from build123d import *

# Parameters (mm, degrees)
SKETCH1_R           = 12.3
SKETCH1_R_2         = 11.9
SKETCH1_R_3         = 10.3
SKETCH1_R_4         = 10.95
SKETCH1_R_5         = 12.35
SKETCH1_R_6         = 9
BOSS_EXTRUDE4_DEPTH = 59
SKETCH4_R           = 8.15
SKETCH4_R_2         = 11.5
SKETCH4_R_3         = 10.1
SKETCH4_R_4         = 11.45
SKETCH4_R_5         = 9.45
SKETCH4_R_6         = 11.05
CUT_EXTRUDE2_DEPTH  = 57
BOSS_EXTRUDE5_DEPTH = 2


with BuildPart() as part:
    # Sketch1 → Boss-Extrude4 (new body)
    with BuildSketch(Plane(origin=(0, 0, 0), x_dir=(1, 0, 0), z_dir=(0, 1, 0))):
        with Locations((35.512781465, 27.639016147)):
            Circle(SKETCH1_R)
        with Locations((36.005267937, -1.447561772)):
            Circle(SKETCH1_R_2)
        with Locations((51.661033243, 13.068619292)):
            Circle(SKETCH1_R_3)
        with Locations((18.919707674, 12.591428229)):
            Circle(SKETCH1_R_4)
        with Locations((6.200754384, 31.090907335)):
            Circle(SKETCH1_R_5)
        with Locations((22.571970647, 43.529254056)):
            Circle(SKETCH1_R_6)
    extrude(amount=BOSS_EXTRUDE4_DEPTH)

    # Sketch4 → Cut-Extrude2 (cut)
    with BuildSketch(Plane(origin=(0, 59, 0), x_dir=(1, 0, 0), z_dir=(0, 1, 0))):
        with Locations(Location((22.611280457, 43.589861599, 0), (0, 0, 270))):
            Circle(SKETCH4_R)
        with Locations(Location((6.240064194, 31.151514878, 0), (0, 0, 270))):
            Circle(SKETCH4_R_2)
        with Locations(Location((18.959017484, 12.652035772, 0), (0, 0, 270))):
            Circle(SKETCH4_R_3)
        with Locations(Location((35.552091275, 27.69962369, 0), (0, 0, 270))):
            Circle(SKETCH4_R_4)
        with Locations(Location((51.700343053, 13.129226835, 0), (0, 0, 270))):
            Circle(SKETCH4_R_5)
        with Locations(Location((36.044577747, -1.386954229, 0), (0, 0, 270))):
            Circle(SKETCH4_R_6)
    extrude(amount=-CUT_EXTRUDE2_DEPTH, mode=Mode.SUBTRACT)

    # Sketch5 → Boss-Extrude5 (add)
    with BuildSketch(Plane(origin=(0, 59, 0), x_dir=(1, 0, 0), z_dir=(0, 1, 0))):
        Polygon((40.81243907, -1.58402798), (51.520532369, 9.252965923), (56.778337624, 3.7224031), (58.688878923, 5.538719884), (16.370888419, 50.052027945), (14.460347121, 48.235711161), (17.926333207, 44.589921166), (6.147145479, 32.668939341), (-1.681518051, 40.404484846), (-3.988115938, 38.070120871), (44.470030089, -9.811639827), (46.776627976, -7.477275852), align=None)
        Polygon((36.463308943, 25.091308361), (47.227733247, 13.768461283), (36.382771282, 2.792951133), (25.275141449, 13.768461283), align=None, mode=Mode.SUBTRACT)
        Polygon((21.642995472, 40.680450739), (32.86204414, 28.879394887), (21.559056386, 17.440345379), (9.982307257, 28.879394887), align=None, mode=Mode.SUBTRACT)
    extrude(amount=BOSS_EXTRUDE5_DEPTH)


solid = part.part
Build history of the part. All positions in model axes, mm. A direction names the side the tool comes from. Coordinates: 2 decimals unless noted, no trailing zeros. Order: outer loops, then holes, each group sorted by start corner. A loop starts at its lowest first (then second) coordinate and runs counter-clockwise, first axis right, second up. Notation, with made-up numbers: (41.25, 0.5) - (48.25, 0.5) arc R21 cw to (48.25, 33.5) - close; hole circle Ø8 at (-17, -15.5). An arc over 180 degrees is marked (long way). Write item = value, one per line. Start each with the question number.
1) Wall check: line 1 along X through (y, z) = (26.5, -37); line 2 along X through (y, z) = (35, -40.5); line 3 along X through (y, z) = (6, -15). Give the ranges that are in metal, low to high. Write a range as from..to.
2) 3-axis set-ups, long thin cutter, end or side, ignore diameter. For faces 4 (the face through (15.85, 59.99, -23.08)), 5 (the face through (44, 59, -36)), 6 (the face through (19.902, 59.986, -14.464)): which of +Z, -Z, +X, -X, +Y, -Y reach the whole face in a straight line?
3) Saw through at C-C on y = 36. Count the separate pieces of the cut face and the enclosed holes in it, then the cut area to 3 significant figures.
4) Saw through at B-B on x = 50. Write the cut outline in (y, z) (3 decimals).
5) Two-plate mould, pull along X, no slides. Class faces 1 (the face through (10.788, 29.087, -5.258)), 2 (the face through (57.7, 60, -4.6)), 3 (the face through (14, 59, -44)): pulls with the +X half, pulls with the -X half, needs draft (parallel to the pull), parting line crosses it, or undercut.
6) Saw through at A-A on z = -12.5. Write the cut outline in (x, y), then the cut area to 3 significant figures.
7) Saw through at D-D on x = 34.5. Write the cut outline in (y, z), then the cut area to 3 significant figures.
8) Flat gauge pins, fed straight in: pin 1 Ø15 at (x, z) = (21, -2.5) entering from +Y; pin 2 Ø3 at (y, z) = (11, -14) entering from -X; pin 3 Ø6 at (x, z) = (23, -21.5) entering from -Y; pin 4 Ø6 at (x, y) = (13, 47.5) entering from +Z. Where does each tip first touch, or does it go through?
From the geometry:
q1.line_1 = -4.64..-3.66, 16.14..17.82, 27.41..28.87, 42.23..43.49
q1.line_2 = -1.8..-0.46, 12.94..15.07, 30.15..31.05
q1.line_3 = 8.24..9.14, 28.78..29.6, 41.54..42.44, 60.96..61.78
q2.face_4 = +Y
q2.face_5 = -Z, +X, +Y
q2.face_6 = +Z, -X, +Y
q3.separate_pieces = 1
q3.enclosed_holes = 8
q3.area = 320 mm^2
q4.outline = (0, -23.234) - (59, -23.234) - (59, -22.425) - (2, -22.425) - (2, -3.833) - (59, -3.833) - (59, -2.903) - (0, -2.903) - close; (59, -14.678) - (61, -14.678) - (61, -7.714) - (59, -7.714) - close
q5.face_1 = undercut
q5.face_2 = pulls with the +X half
q5.face_3 = needs draft
q6.outline = (7.97, 0) - (29.87, 0) - (29.87, 59) - (29.06, 59) - (29.06, 2) - (8.86, 2) - (8.86, 59) - (7.97, 59) - close; (21.89, 59) - (26.56, 59) - (26.56, 61) - (21.89, 61) - close; (41.38, 0) - (61.95, 0) - (61.95, 59) - (61.13, 59) - (61.13, 2) - (42.27, 2) - (42.27, 59) - (41.38, 59) - close; (45.97, 59) - (52.07, 59) - (52.07, 61) - (45.97, 61) - close
q6.area = 301 mm^2
q7.outline = (0, -39.9) - (59, -39.9) - (59, -39.1) - (2, -39.1) - (2, -16.3) - (59, -16.3) - (59, -15.38) - (0, -15.38) - close; (0, -10.36) - (59, -10.36) - (59, -9.55) - (2, -9.55) - (2, 12.33) - (59, 12.33) - (59, 13.25) - (0, 13.25) - close; (59, -30.98) - (61, -30.98) - (61, -23.1) - (59, -23.1) - close; (59, -4.65) - (61, -4.65) - (61, -0.04) - (59, -0.04) - close
q7.area = 317 mm^2
q8.pin_1 = 59
q8.pin_2 = 7.97
q8.pin_3 = 0
q8.pin_4 = -2.04
